Build history of the part. All positions in model axes, mm. Face numbers are marked on the shaded views. A direction names the side the tool comes from. Round coordinates to 2 decimals unless told otherwise and drop trailing zeros. Write each loop counter-clockwise with the first axis right and the second up, starting at its lowest first coordinate (ties: lowest second). Pieces come first, ordered by that corner, then holes.
1) Pull direction Z, two halves, no side cores. Call the marked faces 6, 7 and 8: +Z half, -Z half, draft (parallel to the pull), parting line (faces both ways), or undercut.
2) Wall check: probe 1 along X at (y, z) = (-12.5, 11.75); probe 2 along Z at (x, y) = (36.5, 0); probe 3 along Y at (x, z) = (18, 10.5). Give the ranges that are in metal, low to high.
3) Saw through at B-B (y = -12.5). Write the cut outline in (x, z).
4) Saw through at A-A (x = 0). Write the cut outline in (y, z).
5) Saw through at D-D (x = 18). Write the cut outline in (y, z), plus the area to 3 significant figures.
6) Which spindle directions (+Z, -Z, +X, -X, +Y, -Y) get a long thin tool onto all of the face, cutting with end or side? Do the marked faces 1, 2, 3, 4 and 5. Say none if no direction does.
7) Saw through at C-C (z = 3.75). State how many separate pieces and enclosed holes the cut face has, plus the area to 3 significant figures.
8) Flat gauge pins, fed straight in: pin 1 (12 mm diameter, centred on x = 26, y = -31.5, fed in from +Z); pin 2 (1.1 mm diameter, centred on x = -15, z = 4, fed in from +Y); pin 3 (1.8 mm diameter, centred on y = 15.5, z = 8, fed in from -X); pin 4 (1.9 mm diameter, centred on y = 0, z = 10.5, fed in from -X). Where does each tip first touch, or does it go through?
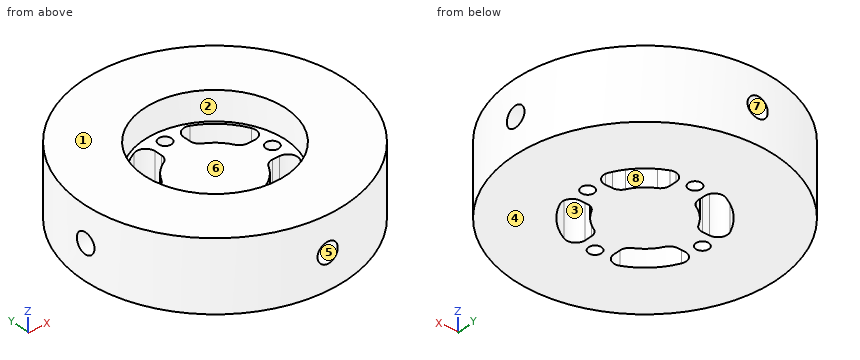
Autodesk Inventor part; units mm, degrees
sketch "Sketch1" plane through (0, 0, 0) normal (0, 0, 1) x (1, 0, 0)
  circle A0 centre (0, 0) radius 40.7
  dimension "d0" = 81.4
extrude "Extrusion1" add sketch "Sketch1" along normal blind 21.75
sketch "Sketch2" plane through (0, 0, 21.75) normal (0, 0, 1) x (1, 0, 0)
  circle A0 centre (0, 0) radius 22
  dimension "d3" = 44
extrude "Extrusion2" cut sketch "Sketch2" against normal blind 9
sketch "Sketch3" plane through (0, 0, 12.75) normal (0, 0, 1) x (1, 0, 0)
  circle A0 centre (0, 18) radius 2
  circle A1 centre (-18, 0) radius 2
  circle A2 centre (0, -18) radius 2
  circle A3 centre (18, 0) radius 2
  point P0 (0, 0)
  dimension "d6" = 4
  dimension "d7" = 18
  dimension "d10" = 360
extrude "Extrusion3" cut sketch "Sketch3" against normal blind 12.75
sketch "Sketch4" plane through (0, 0, 12.75) normal (0, 0, 1) x (1, 0, 0)
  arc A0 (-4.5165, 17.448) -> (-8.8542, 19.2414) centre (-7.5165, 16.3345) ccw
  arc A1 (-8.8542, 19.2414) -> (-19.0977, 9.16) centre (0, 0) ccw
  arc A2 (-14.1333, 4.5) -> (-11.4833, 6.0938) centre (-14.1333, 7.5) ccw
  line L0 (-4.5, 14.1333) -> (-4.5, 16.3631)
  arc A3 (-4.5, 16.3631) -> (-8.75, 19.0902) centre (-7.5, 16.3631) ccw
  arc A4 (-6.0938, 11.4833) -> (-4.5, 14.1333) centre (-7.5, 14.1333) ccw
  arc A5 (-6.0938, 11.4833) -> (-11.4833, 6.0938) centre (0, 0) ccw
  arc A6 (-8.8542, 19.2414) -> (-19.2547, 8.8254) centre (0, 0) ccw
  arc A7 (-8.75, 19.0902) -> (-19.0902, 8.75) centre (0, 0) ccw
  arc A8 (-19.0902, 8.75) -> (-16.3631, 4.5) centre (-16.3631, 7.5) ccw
  line L1 (-16.3631, 4.5) -> (-14.1333, 4.5)
  arc A9 (-11.4833, -6.0938) -> (-14.1333, -4.5) centre (-14.1333, -7.5) ccw
  arc A10 (-4.5, -14.1333) -> (-6.0938, -11.4833) centre (-7.5, -14.1333) ccw
  arc A11 (-11.4833, -6.0938) -> (-6.0938, -11.4833) centre (0, 0) ccw
  line L2 (-14.1333, -4.5) -> (-16.3631, -4.5)
  line L3 (-4.5, -16.3631) -> (-4.5, -14.1333)
  arc A12 (-16.3631, -4.5) -> (-19.0902, -8.75) centre (-16.3631, -7.5) ccw
  arc A13 (-17.448, -4.5165) -> (-19.2414, -8.8542) centre (-16.3345, -7.5165) ccw
  arc A14 (-8.75, -19.0902) -> (-4.5, -16.3631) centre (-7.5, -16.3631) ccw
  arc A15 (-19.0902, -8.75) -> (-8.75, -19.0902) centre (0, 0) ccw
  arc A16 (-19.2414, -8.8542) -> (-9.16, -19.0977) centre (0, 0) ccw
  arc A17 (-19.2414, -8.8542) -> (-8.8254, -19.2547) centre (0, 0) ccw
  arc A18 (6.0938, -11.4833) -> (4.5, -14.1333) centre (7.5, -14.1333) ccw
  arc A19 (14.1333, -4.5) -> (11.4833, -6.0938) centre (14.1333, -7.5) ccw
  arc A20 (6.0938, -11.4833) -> (11.4833, -6.0938) centre (0, 0) ccw
  line L4 (4.5, -14.1333) -> (4.5, -16.3631)
  line L5 (16.3631, -4.5) -> (14.1333, -4.5)
  arc A21 (4.5, -16.3631) -> (8.75, -19.0902) centre (7.5, -16.3631) ccw
  arc A22 (4.5165, -17.448) -> (8.8542, -19.2414) centre (7.5165, -16.3345) ccw
  arc A23 (19.0902, -8.75) -> (16.3631, -4.5) centre (16.3631, -7.5) ccw
  arc A24 (8.75, -19.0902) -> (19.0902, -8.75) centre (0, 0) ccw
  arc A25 (8.8542, -19.2414) -> (19.0977, -9.16) centre (0, 0) ccw
  arc A26 (8.8542, -19.2414) -> (19.2547, -8.8254) centre (0, 0) ccw
  arc A27 (11.4833, 6.0938) -> (14.1333, 4.5) centre (14.1333, 7.5) ccw
  arc A28 (4.5, 14.1333) -> (6.0938, 11.4833) centre (7.5, 14.1333) ccw
  arc A29 (11.4833, 6.0938) -> (6.0938, 11.4833) centre (0, 0) ccw
  line L6 (14.1333, 4.5) -> (16.3631, 4.5)
  line L7 (4.5, 16.3631) -> (4.5, 14.1333)
  arc A30 (16.3631, 4.5) -> (19.0902, 8.75) centre (16.3631, 7.5) ccw
  arc A31 (17.448, 4.5165) -> (19.2414, 8.8542) centre (16.3345, 7.5165) ccw
  arc A32 (8.75, 19.0902) -> (4.5, 16.3631) centre (7.5, 16.3631) ccw
  arc A33 (19.0902, 8.75) -> (8.75, 19.0902) centre (0, 0) ccw
  arc A34 (19.2414, 8.8542) -> (9.16, 19.0977) centre (0, 0) ccw
  arc A35 (19.2414, 8.8542) -> (8.8254, 19.2547) centre (0, 0) ccw
  point P0 (41.0732, 32.7294)
  point P1 (-17.4931, 4.4714)
  point P2 (-16.3796, 7.4714)
  point P3 (-7.4714, -16.3796)
  point P4 (-4.4714, -17.4931)
  point P5 (16.3796, -7.4714)
  point P6 (17.4931, -4.4714)
  point P7 (7.4714, 16.3796)
  point P8 (4.4714, 17.4931)
  dimension "d16" = 360
extrude "Extrusion4" cut sketch "Sketch4" against normal blind 12.75
ref_plane "Work Plane1" through (40.7, 0, 0) normal (1, 0, 0) x (0, 1, 0)
sketch "Sketch6" plane through (40.7, 0, 0) normal (1, 0, 0) x (0, 1, 0)
  circle A0 centre (0, 10.875) radius 3.175
  point P0 (0, 0)
  dimension "d24" = 6.35
extrude "Extrusion5" cut sketch "Sketch6" against normal blind 12.7
pattern_circular "Circular Pattern1" count 4 over 360 about axis through (0, 0, -10) along (0, 0, 1) of "Extrusion5"
properties part number "MotorHousing"
Evaluation:
1. face 6: +Z half
1. face 7: undercut
1. face 8: draft
2. probe 1: x = -38.73 to -16.87, -4.98 to 4.98, 16.87 to 38.73
2. probe 2: z = 0 to 7.7, 14.05 to 21.75
2. probe 3: y = -36.5 to -10.82, -4.99 to -2, 2 to 4.99, 10.82 to 36.5
3. outline: (-38.73, 0) - (-16.87, 0) - (-16.87, 12.75) - (-18.1, 12.75) - (-18.1, 21.75) - (-38.73, 21.75) - close; (-4.98, 0) - (4.98, 0) - (4.98, 12.75) - (-4.98, 12.75) - close; (16.87, 0) - (38.73, 0) - (38.73, 21.75) - (18.1, 21.75) - (18.1, 12.75) - (16.87, 12.75) - close
4. outline: (-40.7, 0) - (-20, 0) - (-20, 12.75) - (-22, 12.75) - (-22, 21.75) - (-40.7, 21.75) - (-40.7, 14.05) - (-28, 14.05) - (-28, 7.7) - (-40.7, 7.7) - close; (-16, 0) - (16, 0) - (16, 12.75) - (-16, 12.75) - close; (20, 0) - (40.7, 0) - (40.7, 7.7) - (28, 7.7) - (28, 14.05) - (40.7, 14.05) - (40.7, 21.75) - (22, 21.75) - (22, 12.75) - (20, 12.75) - close
5. outline: (-36.5, 0) - (-10.82, 0) - (-10.82, 12.75) - (-12.65, 12.75) - (-12.65, 21.75) - (-36.5, 21.75) - close; (-4.99, 0) - (-2, 0) - (-2, 12.75) - (-4.99, 12.75) - close; (2, 0) - (4.99, 0) - (4.99, 12.75) - (2, 12.75) - close; (10.82, 0) - (36.5, 0) - (36.5, 21.75) - (12.65, 21.75) - (12.65, 12.75) - (10.82, 12.75) - close
5. area: 1,160 mm2
6. face 1: +Z, +X, -X, +Y, -Y
6. face 2: +Z
6. face 3: +Z, -Z
6. face 4: -Z, +X, -X, +Y, -Y
6. face 5: -Y
7. separate pieces: 1
7. enclosed holes: 8
7. area: 4,630 mm2
8. pin 1: stops at z = 21.75
8. pin 2: stops at y = 38.05
8. pin 3: stops at x = -37.99
8. pin 4: stops at x = -28
